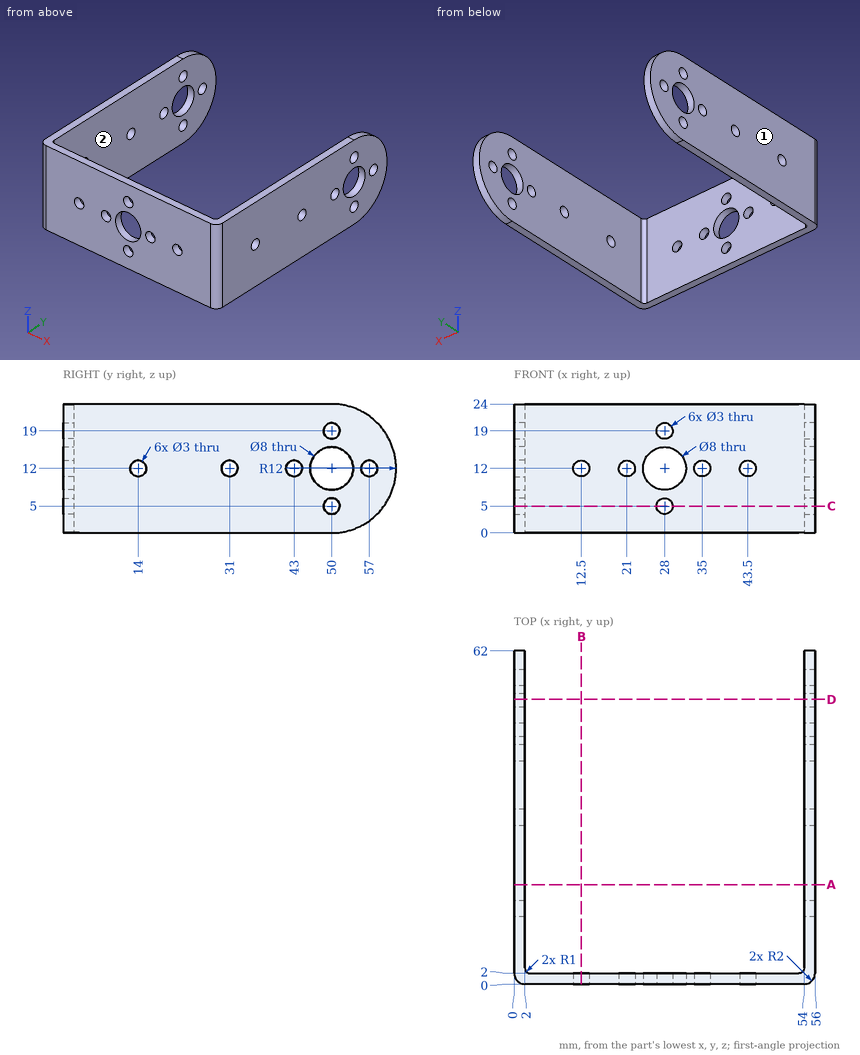
Could you check a few things on this drawing? It's one solid part, dimensions in mm from its lowest x, y, z. A direction names the side the tool comes from. Coordinates: 2 decimals unless noted, no trailing zeros. Order: outer loops, then holes, each group sorted by start corner. A loop starts at its lowest first (then second) coordinate and runs counter-clockwise, first axis right, second up. Notation, with made-up numbers: M 31,9 L 56,9 A26 cw 56,32 Z; hole C -40,30 d2. An arc over 180 degrees is marked long. Answer as a JSON object with one key per item and string values. Group by question number.
(1) Suppose I cut it at A-A, the plane y = 18.5. Please give me the cut outline in (x, z).
(2) Suppose I cut it at B-B, the plane x = 12.5. Please give me the cut outline in (y, z).
(3) Suppose I cut it at D-D, the plane y = 53. Please give me the cut outline in (x, z).
(4) Which directions (+Z, -Z, +X, -X, +Y, -Y) give clear straight access to the entire face, cutting with the end or side of a thin tool? Please do the marked faces 1 and 2.
(5) I need wall thicknesses on probe 1 along X at (y, z) = (26.5, 22); probe 2 along X at (y, z) = (1.15, 12); probe 3 along Y at (x, z) = (54.55, 12). Which ranges of each line are inside material? Lowest first, please.
(6) For pin 1 (6 mm diameter, centred on x = 50, z = 6, fed in from +Y), with a flat end and sliding along its axis, tell me the tip position at first contact or that it passes through.
(7) Suppose I cut it at C-C, the plane z = 5. Please give me the cut outline in (x, y), then the cut area to 3 significant figures.
Values found:
{
 "1": {"outline": "M 0,0 L 2,0 L 2,24 L 0,24 Z; M 54,0 L 56,0 L 56,24 L 54,24 Z"},
 "2": {"outline": "M 0,0 L 2,0 L 2,10.5 L 0,10.5 Z; M 0,13.5 L 2,13.5 L 2,24 L 0,24 Z"},
 "3": {"outline": "M 0,0.38 L 2,0.38 L 2,9.35 L 0,9.35 Z; M 0,14.65 L 2,14.65 L 2,23.62 L 0,23.62 Z; M 54,0.38 L 56,0.38 L 56,9.35 L 54,9.35 Z; M 54,14.65 L 56,14.65 L 56,23.62 L 54,23.62 Z"},
 "4": {"face 1": "+Z, -Z, -X, +Y, -Y", "face 2": "+Z, -Z, +Y"},
 "5": {"probe 1": "x = 0 to 2, 54 to 56", "probe 2": "x = 0.19 to 11, 14 to 19.5, 22.5 to 24, 32 to 33.5, 36.5 to 42, 45 to 55.81", "probe 3": "y = 0.08 to 12.5, 15.5 to 29.5, 32.5 to 41.5, 44.5 to 46, 54 to 55.5, 58.5 to 62"},
 "6": {"pin 1": "stops at y = 2"},
 "7": {"outline": "M 0,2 A2 ccw 2,0 L 26.5,0 L 26.5,2 L 3,2 A1 cw 2,3 L 2,48.5 L 0,48.5 Z; M 0,51.5 L 2,51.5 L 2,59.75 L 0,59.75 Z; M 29.5,0 L 54,0 A2 ccw 56,2 L 56,48.5 L 54,48.5 L 54,3 A1 cw 53,2 L 29.5,2 Z; M 54,51.5 L 56,51.5 L 56,59.75 L 54,59.75 Z", "area": "324 mm^2"}
}
